from build123d import *

# Parameters (mm, degrees)
F3_DEPTH = 12.701


with BuildPart() as f1:
    # F0 (on Front) → F1 (revolve)
    with BuildSketch(Plane.XZ):
        with BuildLine():
            Line((0, -6.35), (0, 0))
            Line((0, 0), (0, 6.35))
            Line((0, 6.35), (-11.7475, 6.35))
            Line((-11.7475, 6.35), (-11.7475, 1.5875))
            ThreePointArc((-11.7475, 1.5875), (-10.624968, 1.122532), (-10.16, 0))
            ThreePointArc((-10.16, 0), (-10.624968, -1.122532), (-11.7475, -1.5875))
            Line((-11.7475, -1.5875), (-11.7475, -6.35))
            Line((-11.7475, -6.35), (0, -6.35))
        make_face()
    revolve(axis=Axis((0, 0, 3.175), (0, 0, 1)))

    # F2 (on face) → F3 (cut, through all)
    with BuildSketch(Plane.XY.offset(6.35)):
        with BuildLine():
            ThreePointArc((-2.846846, 1.54381), (-0.796358, -3.13906), (3.2385, 0))
            ThreePointArc((3.2385, 0), (3.13906, 0.796358), (2.846846, 1.54381))
            Line((2.846846, 1.54381), (-2.846846, 1.54381))
        make_face()
    extrude(amount=-F3_DEPTH, mode=Mode.SUBTRACT)


solid = f1.part
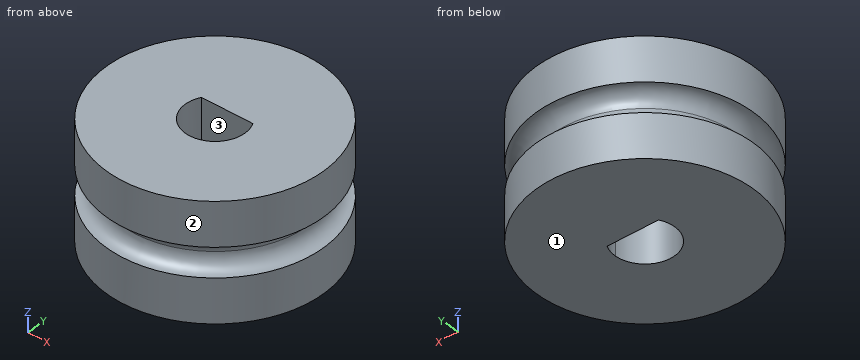
Input: part model. Units: mm. Frame: model coordinates. Face numbers are marked on the shaded views. Coordinates: 2 decimals unless noted, no trailing zeros. Loops run counter-clockwise (first coordinate to the right, second up) from the corner with the lowest first, then second, coordinate; pieces in that order, holes last.
Q1. Material intervals for line 1 (X direction, y = 0, z = 3.5); line 2 (Y direction, x = 0, z = 3.75); line 3 (Y direction, x = 1.75, z = 0.75), sorted ascending.
Q2. Draft query along Y for the marked faces 1, 2 and 3. Return one class per face: +Y half, -Y half, draft (parallel to the pull), parting line (faces both ways), or undercut.
Q3. Cut plane A-A (z = 3.5). Output: boundary loops of the cut face in (x, y) (1 decimal), then the cut area to 3 significant figures.
Q4. Contact query for flat-ended pins moving along their axis: pin 1 (1.5 mm diameter, centred on y = 0.5, z = -2, fed in from +X); pin 2 (2 mm diameter, centred on x = -9, z = 4, fed in from -Y); pin 3 (1.5 mm diameter, centred on y = 8.5, z = -2.5, fed in from +X). Output: stop coordinate, or through.
Working result:
1. line 1: x = -11.75 to -3.24, 3.24 to 11.75
1. line 2: y = -11.75 to -3.24, 1.54 to 11.75
1. line 3: y = -10.2 to -2.72, 1.54 to 10.2
2. face 1: draft
2. face 2: parting line
2. face 3: undercut
3. outline: circle Ø23.5 at (0, 0); hole (-2.8, 1.5) arc R3.2 ccw (long way) to (3.2, 0) arc R3.2 ccw to (2.8, 1.5) - close
3. area: 407 mm2
4. pin 1: stops at x = 11.75
4. pin 2: stops at y = -8.6
4. pin 3: stops at x = 8.83
